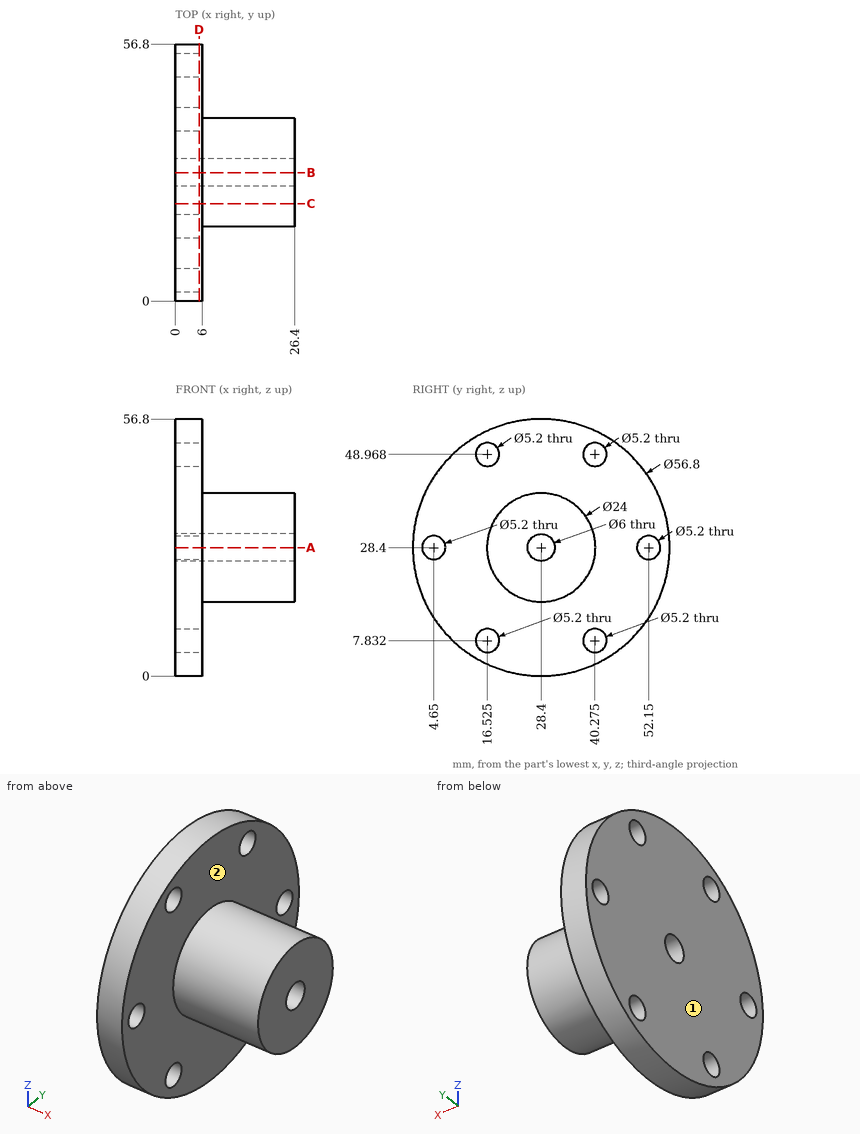
Part print with two shaded views. Sizes in mm from the minimum x, y, z corner. A direction names the side the tool comes from. Round coordinates to 2 decimals unless told otherwise and drop trailing zeros. Loops run counter-clockwise (first coordinate to the right, second up) from the corner with the lowest first, then second, coordinate; pieces in that order, holes last. Notation, with made-up numbers: (46, -31.5) - (50, -31.5) arc R19 cw to (50, -14.5) - close; hole circle Ø6 at (-1, -27). An arc over 180 degrees is marked (long way). Answer as a JSON object with one key per item and string values.
Item 1: Band-saw the part on A-A on z = 28.4. List the corners of the cut face in (x, y).
Output:
{"outline": "(0, 0) - (6, 0) - (6, 2.05) - (0, 2.05) - close; (0, 7.25) - (6, 7.25) - (6, 16.4) - (26.4, 16.4) - (26.4, 25.4) - (0, 25.4) - close; (0, 31.4) - (26.4, 31.4) - (26.4, 40.4) - (6, 40.4) - (6, 49.55) - (0, 49.55) - close; (0, 54.75) - (6, 54.75) - (6, 56.8) - (0, 56.8) - close"}
Item 2: Band-saw the part on C-C on y = 21.5. List the corners of the cut face in (x, z).
Output:
{"outline": "(0, 0.85) - (6, 0.85) - (6, 18.58) - (26.4, 18.58) - (26.4, 38.22) - (6, 38.22) - (6, 55.95) - (0, 55.95) - close"}
Item 3: Band-saw the part on B-B on y = 28.4. List the corners of the cut face in (x, z).
Output:
{"outline": "(0, 0) - (6, 0) - (6, 16.4) - (26.4, 16.4) - (26.4, 25.4) - (0, 25.4) - close; (0, 31.4) - (26.4, 31.4) - (26.4, 40.4) - (6, 40.4) - (6, 56.8) - (0, 56.8) - close"}
Item 4: Pin check, flat tips, straight feed: pin 1 (8.5 mm diameter, centred on y = 16.52, z = 48.97, fed in from +X); pin 2 (5 mm diameter, centred on x = 19.5, z = 18, fed in from +Y); pin 3 (10 mm diameter, centred on x = 3.5, z = 46, fed in from +Y); pin 4 (4 mm diameter, centred on y = 40.28, z = 48.97, fed in from +X). Stop position of each tip, or through.
Output:
{"pin 1": "x = 6", "pin 2": "y = 37.43", "pin 3": "y = 53.85", "pin 4": "through"}
Item 5: Wall check: L1, parallel to Y at x = 7.75, z = 28.4; L2, parallel to Z at x = 4.5, y = 15.5; L3, parallel to X at y = 21, z = 10.5. Give the ranges that are in metal, low to high.
Output:
{"L1": "16.4 to 25.4, 31.4 to 40.4", "L2": "3.1 to 5.44, 10.22 to 46.58, 51.36 to 53.7", "L3": "0 to 6"}
Item 6: Band-saw the part on D-D on x = 5.25. List the corners of the cut face in (y, z) (3 decimals), plus the area to 3 significant figures.
Output:
{"outline": "circle Ø56.8 at (28.4, 28.4); hole circle Ø5.2 at (4.65, 28.4); hole circle Ø5.2 at (16.525, 7.832); hole circle Ø5.2 at (16.525, 48.968); hole circle Ø6 at (28.4, 28.4); hole circle Ø5.2 at (40.275, 7.832); hole circle Ø5.2 at (40.275, 48.968); hole circle Ø5.2 at (52.15, 28.4)", "area": "2,380 mm2"}
Item 7: Tool access for the marked faces 1 and 2: list every direction of +Z, -Z, +X, -X, +Y, -Y with a clear straight run to the whole face (end or side of a thin tool).
Output:
{"face 1": "+Z, -Z, -X, +Y, -Y", "face 2": "+X"}
